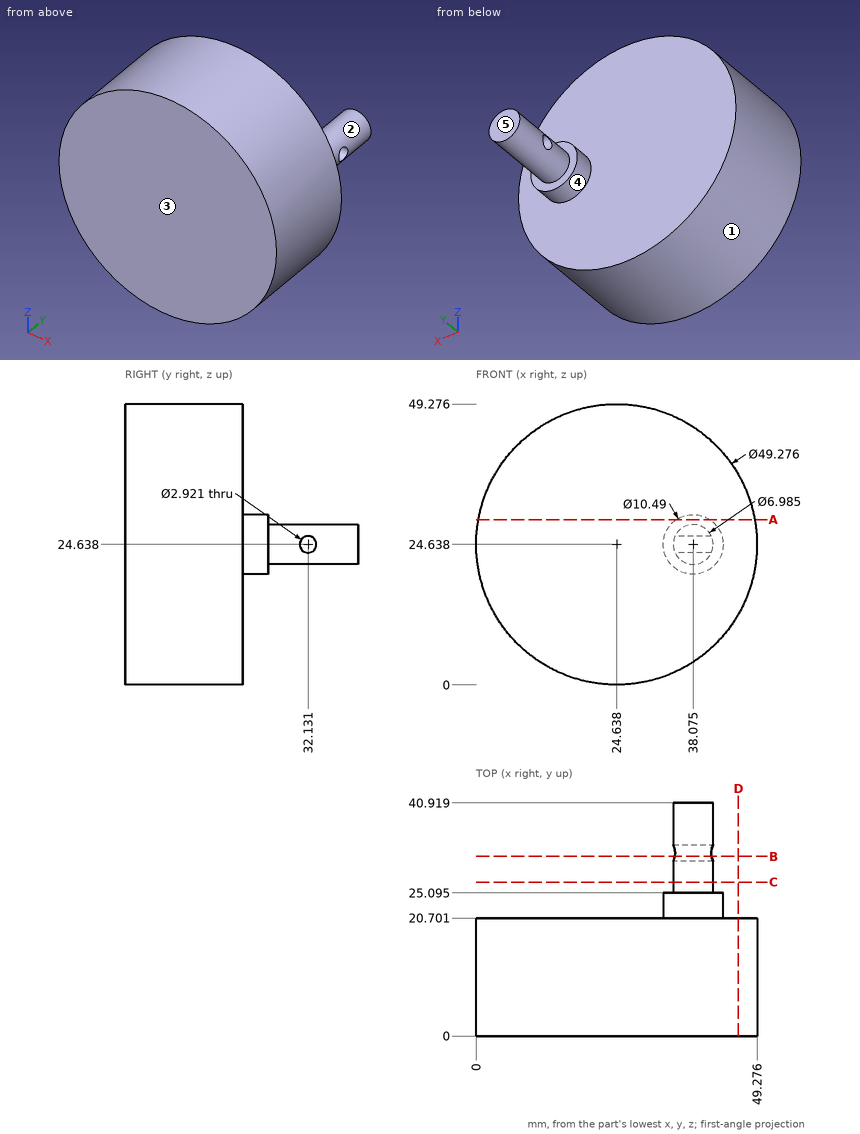
Input: dimensioned drawing with shaded views. Units: mm. Origin: part minimum x, y, z. A direction names the side the tool comes from. Round coordinates to 2 decimals unless told otherwise and drop trailing zeros. Loops run counter-clockwise (first coordinate to the right, second up) from the corner with the lowest first, then second, coordinate; pieces in that order, holes last. Notation, with made-up numbers: M -23,33.25 L 9,33.25 A25 ccw 9,49.25 Z; hole C -18.75,-2.5 d7. An arc over 180 degrees is marked long. One line per question, with ' | ' between items.
(1) Cut plane C-C on y = 27. Return the cut outline in (x, z) (1 decimal), plus the area to 3 significant figures.
Check result:
outline: C 38.1,24.6 d7 | area: 38.3 mm2
(2) Cut plane A-A on z = 29. Return the cut outline in (x, y) (1 decimal), plus the area to 3 significant figures.
Check result:
outline: M 0.4,0 L 48.9,0 L 48.9,20.7 L 41,20.7 L 41,25.1 L 35.2,25.1 L 35.2,20.7 L 0.4,20.7 Z | area: 1,030 mm2
(3) Contact query for flat-ended pins moving along their axis: P1, Ø1, axis at x = 13, y = 11.5, coming from the -Z side; P2, Ø3, axis at x = 42, z = 43.5, coming from the +Y side; P3, Ø3.5, axis at y = 32.131, z = 24.638, coming from the -X side; P4, Ø2, axis at y = 35.5, z = 19.5, coming from the -X side. Output: stop coordinate, or through.
Check result:
P1: stops at z = 2.66 | P2: stops at y = 20.7 | P3: stops at x = 34.58 | P4: passes through
(4) Pull-direction query (Y, two-part tool) for the marked faces 3, 4 and 5; classes: +Y half, -Y half, draft (parallel to the pull), parting line (faces both ways), or undercut.
Check result:
face 3: -Y half | face 4: draft | face 5: +Y half
(5) Access query for the marked faces 1 and 2. Directions: +Z, -Z, +X, -X, +Y, -Y. A direction counts if a zero-diameter tool reaches every point of the face in a straight line with its end or side. Return the directions, or none.
Check result:
face 1: +Y, -Y | face 2: +Y
(6) Cut plane B-B on y = 31.5. Return the cut outline in (x, z) (1 decimal).
Check result:
outline: M 34.8,23.3 A3.5 ccw 41.3,23.3 Z; M 34.8,26 L 41.3,26 A3.5 ccw Z
(7) Cut plane D-D on x = 46. Return the cut outline in (y, z).
Check result:
outline: M 0,12.36 L 20.7,12.36 L 20.7,36.91 L 0,36.91 Z
(8) Material intervals for line 1 along Y through (x, z) = (20.5, 47.5); line 2 along X through (y, z) = (16.5, 14.5) (1 decimal); line 3 along X through (y, z) = (16.5, 15), sorted ascending. Write a range as from..to.
Check result:
line 1: y = 0..20.7 | line 2: x = 2.2..47.1 | line 3: x = 1.96..47.31
